Geometry check sheet. Reference: the model listing, model coordinates, mm. Round coordinates to 2 decimals unless told otherwise and drop trailing zeros. Order: outer loops, then holes, each group sorted by start corner. A loop starts at its lowest first (then second) coordinate and runs counter-clockwise, first axis right, second up.
(1) Draft check along X on faces 1 (the face through (-3.688, 28.086, 1.519)), 2 (the face through (0, 0, -16.51)), 3 (the face through (0, 0, -19.05)), 4 (the face through (-4.018, 30.604, -1.964)). Enter one of: pulls with the +X half, pulls with the -X half, needs draft (parallel to the pull), parting line crosses it, or undercut.
(2) Gauge pin test, flat ends, axial feed: P1, Ø6, axis at x = -14, z = 4.5, coming from the -Y side; P2, Ø1, axis at x = -3.5, z = 8.5, coming from the +Y side; P3, Ø6, axis at y = 17, z = 13.5, coming from the +X side. Record the tip position at first contact, or that the pin passes through.
(3) Cross-section at A-A on x = 0. Enter the section's corners in (y, z), and give its area (3 significant figures).
(4) Thickness scan on L1, parallel to Y at x = 0, z = -1.5; L2, parallel to Z at x = -5, y = 26; L3, parallel to X at y = 11, z = -0.5. Record the ranges inside material, lowest first.
from build123d import *

# Parameters (mm, degrees)
F0_R     = 30.8666383599
F1_DEPTH = 19.05
F2_T     = -2.54


# Not quite as in the source:
# - a fillet or chamfer that OpenCascade refuses, or shapes differently, is made with other operations: its cross-section is extruded or revolved along the edge and cut away or added


with BuildPart() as f1:
    # F0 (on Top) → F1 (new body, symmetric)
    with BuildSketch(Plane.XY):
        Circle(F0_R)
    extrude(amount=F1_DEPTH, both=True)

    # F2
    f2_openings = [f1.faces().sort_by_distance(p)[0] for p in [
        (0, 0, 19.05),
    ]]
    offset(amount=F2_T, openings=f2_openings)

    # F3: fillet of radius 5.08 on 1 edges, made by hand

    # F3_s1 → F3_t2 (revolve, cut)
    with BuildSketch(Plane.XZ):
        with BuildLine():
            ThreePointArc((30.8666383599, 14.6505909488), (30.1860474111, 17.1905909488), (28.3266383599, 19.05))
            Line((28.3266383599, 19.05), (28.3774383599, 19.137988181))
            ThreePointArc((28.3774383599, 19.137988181), (29.5966383599, 19.1516), (30.8666383599, 19.1516))
            Line((30.8666383599, 19.1516), (30.9682383599, 19.05))
            Line((30.9682383599, 19.05), (30.9682383599, 14.6505909488))
            Line((30.9682383599, 14.6505909488), (30.8666383599, 14.6505909488))
        make_face()
    revolve(axis=Axis((0, 0, 19.05), (0, 0, 1)), mode=Mode.SUBTRACT)


solid = f1.part
Found:
1. face 1: undercut
1. face 2: undercut
1. face 3: needs draft
1. face 4: parting line crosses it
2. P1: stops at y = -28.84
2. P2: stops at y = 30.72
2. P3: stops at x = 27.51
3. outline: (-30.87, -19.05) - (30.87, -19.05) - (30.87, 14.65) arc R5.08 ccw to (28.33, 19.05) - (28.33, -16.51) - (-28.33, -16.51) - (-28.33, 19.05) arc R5.08 ccw to (-30.87, 14.65) - close
3. area: 331 mm2
4. L1: y = -30.87 to -28.33, 28.33 to 30.87
4. L2: z = -19.05 to -16.51
4. L3: x = -28.84 to -26.1, 26.1 to 28.84
